from build123d import *

# Parameters (mm, degrees)
SKETCH1_R                                      = 79.248
EXTRUDE1_DEPTH                                 = 3.175
EXTRUDE1_DEPTH_BACK                            = 3.175
SKETCH2_R                                      = 63.5
EXTRUDE2_DEPTH                                 = 10.16
SKETCH4_W                                      = 2.54
SKETCH4_H                                      = 2.3622
SKETCH5_R                                      = 55.88
CUT_EXTRUDE1_DEPTH                             = 10.16
CHAMFER1_SIZE                                  = 1.27
CHAMFER2_SIZE                                  = 0.254
CBORE_FOR_3_SOCKET_HEAD_CAP_SCREW1_D           = 2.794
CBORE_FOR_3_SOCKET_HEAD_CAP_SCREW1_CBORE_D     = 5.15874
CBORE_FOR_3_SOCKET_HEAD_CAP_SCREW1_CBORE_DEPTH = 2.5146
CIRPATTERN1_COUNT                              = 6
F_4_40_TAPPED_HOLE1_D                          = 2.2606
F_4_40_TAPPED_HOLE1_DEPTH                      = 5.08
F_4_40_TAPPED_HOLE1_TIP                        = 0.679152758
M14_CLEARANCE_HOLE1_D                          = 15.5
M14_CLEARANCE_HOLE1_DEPTH                      = 330.2
M14_CLEARANCE_HOLE1_TIP                        = 4.656669797
F_6_32_TAPPED_HOLE1_D                          = 2.7051
F_6_32_TAPPED_HOLE1_DEPTH                      = 4.318
F_6_32_TAPPED_HOLE1_CBORE_D                    = 3.5052
F_6_32_TAPPED_HOLE1_CBORE_DEPTH                = 3.556
F_6_32_TAPPED_HOLE1_TIP                        = 0.81269403
SKETCH21_R                                     = 3.175
SKETCH21_R_2                                   = 1.7526
BOSS_EXTRUDE1_DEPTH                            = 25.4


with BuildPart() as part:
    # Sketch1 → Extrude1 (new body, two sides)
    with BuildSketch(Plane(origin=(0, 0, 0), x_dir=(1, 0, 0), z_dir=(0, 1, 0))) as extrude1_sk:
        Circle(SKETCH1_R)
    extrude(amount=EXTRUDE1_DEPTH)
    extrude(extrude1_sk.sketch, amount=-EXTRUDE1_DEPTH_BACK)

    # Sketch2 → Extrude2 (add)
    with BuildSketch(Plane(origin=(0, 3.175, 0), x_dir=(-1, 0, 0), z_dir=(0, 1, 0))):
        Circle(SKETCH2_R)
    extrude(amount=EXTRUDE2_DEPTH)

    # Sketch4 → Cut-Revolve7 (revolve, cut)
    with BuildSketch(Plane(origin=(0, 0, 0), x_dir=(0, 0, -1), z_dir=(1, 0, 0))):
        with Locations((-62.23, 10.122310801)):
            Rectangle(SKETCH4_W, SKETCH4_H)
        with Locations((-62.23, 6.799968424)):
            Rectangle(SKETCH4_W, SKETCH4_H)
    revolve(axis=Axis((0, -3.175, 0), (0, 1, 0)), mode=Mode.SUBTRACT)

    # Sketch5 → Cut-Extrude1 (cut)
    with BuildSketch(Plane(origin=(0, 13.335, 0), x_dir=(-1, 0, 0), z_dir=(0, 1, 0))):
        Circle(SKETCH5_R)
    extrude(amount=-CUT_EXTRUDE1_DEPTH, mode=Mode.SUBTRACT)

    # Chamfer1
    chamfer1_edges = [part.edges().sort_by_distance(p)[0] for p in [
        (63.5, 13.335, 0),
    ]]
    chamfer(chamfer1_edges, length=CHAMFER1_SIZE)

    # Chamfer2
    chamfer2_edges = [part.edges().sort_by_distance(p)[0] for p in [
        (63.5, 11.303410801, 0),
        (63.5, 8.941210801, 0),
        (63.5, 7.981068424, 0),
        (63.5, 5.618868424, 0),
    ]]
    chamfer(chamfer2_edges, length=CHAMFER2_SIZE)

    # CBORE for _3 Socket Head Cap Screw1 (through all)
    with Locations(Plane(origin=(0, -3.175, 66.675), x_dir=(0, 0, -1), z_dir=(0, -1, 0))):
        with Locations((0, 0)):
            cbore_for_3_socket_head_cap_screw1 = CounterBoreHole(CBORE_FOR_3_SOCKET_HEAD_CAP_SCREW1_D / 2, CBORE_FOR_3_SOCKET_HEAD_CAP_SCREW1_CBORE_D / 2, CBORE_FOR_3_SOCKET_HEAD_CAP_SCREW1_CBORE_DEPTH)

    # CirPattern1: CBORE for _3 Socket Head Cap Screw1 ×6 about axis
    cirpattern1_axis = Axis((0, 0, 0), (0, 1, 0))
    for i in range(1, CIRPATTERN1_COUNT):
        add(cbore_for_3_socket_head_cap_screw1.rotate(cirpattern1_axis, i * 360 / CIRPATTERN1_COUNT), mode=Mode.SUBTRACT)

    # 4-40 Tapped Hole1
    with Locations(Plane(origin=(9.525, 3.175, -36.195), x_dir=(0, 0, 1), z_dir=(0, 1, 0))):
        with Locations((0, 0), (66.675, -26.9875)):
            Hole(F_4_40_TAPPED_HOLE1_D / 2, depth=F_4_40_TAPPED_HOLE1_DEPTH)
            with Locations((0, 0, -(F_4_40_TAPPED_HOLE1_DEPTH + F_4_40_TAPPED_HOLE1_TIP / 2))):  # 118° drill point
                Cone(0, F_4_40_TAPPED_HOLE1_D / 2, F_4_40_TAPPED_HOLE1_TIP, mode=Mode.SUBTRACT)

    # M14 Clearance Hole1
    with Locations(Plane(origin=(-45.367887501, 3.175, 0), x_dir=(0, 0, 1), z_dir=(0, 1, 0))):
        with Locations((0, 0)):
            Hole(M14_CLEARANCE_HOLE1_D / 2, depth=M14_CLEARANCE_HOLE1_DEPTH)
            with Locations((0, 0, -(M14_CLEARANCE_HOLE1_DEPTH + M14_CLEARANCE_HOLE1_TIP / 2))):  # 118° drill point
                Cone(0, M14_CLEARANCE_HOLE1_D / 2, M14_CLEARANCE_HOLE1_TIP, mode=Mode.SUBTRACT)

    # 6-32 Tapped Hole1
    with Locations(Plane(origin=(-19.05, -3.175, 20.574), x_dir=(0, 0, -1), z_dir=(0, -1, 0))):
        with Locations((0, 0), (0, 38.1), (41.148, 38.1), (41.148, 0)):
            CounterBoreHole(F_6_32_TAPPED_HOLE1_D / 2, F_6_32_TAPPED_HOLE1_CBORE_D / 2, F_6_32_TAPPED_HOLE1_CBORE_DEPTH, depth=F_6_32_TAPPED_HOLE1_DEPTH)
            with Locations((0, 0, -(F_6_32_TAPPED_HOLE1_DEPTH + F_6_32_TAPPED_HOLE1_TIP / 2))):  # 118° drill point
                Cone(0, F_6_32_TAPPED_HOLE1_D / 2, F_6_32_TAPPED_HOLE1_TIP, mode=Mode.SUBTRACT)

    # Sketch21 → Boss-Extrude1 (add)
    with BuildSketch(Plane.XZ.offset(3.175)):
        with Locations((19.05, -20.574)):
            Circle(SKETCH21_R)
        with Locations((19.05, -20.574)):
            Circle(SKETCH21_R_2, mode=Mode.SUBTRACT)
        with Locations((-19.05, -20.574)):
            Circle(SKETCH21_R)
        with Locations((-19.05, -20.574)):
            Circle(SKETCH21_R_2, mode=Mode.SUBTRACT)
        with Locations((-19.05, 20.574)):
            Circle(SKETCH21_R)
        with Locations((-19.05, 20.574)):
            Circle(SKETCH21_R_2, mode=Mode.SUBTRACT)
        with Locations((19.05, 20.574)):
            Circle(SKETCH21_R)
        with Locations((19.05, 20.574)):
            Circle(SKETCH21_R_2, mode=Mode.SUBTRACT)
    extrude(amount=BOSS_EXTRUDE1_DEPTH)


solid = part.part
Input: part model. Units: mm. Frame: model coordinates. A direction names the side the tool comes from. Give positions to 0.01 mm unless a question says otherwise; leave off trailing zeros. Order: outer loops, then holes, each group sorted by start corner. A loop starts at its lowest first (then second) coordinate and runs counter-clockwise, first axis right, second up. Notation, with made-up numbers: (75.25, 5) -> (114.25, 5) arc R32 cw to (114.25, 41) -> close; hole circle Ø6 at (87, 31). An arc over 180 degrees is marked (long way). Use one line per item in the form item = value.
1) Line query: probe 1 along X at (y, z) = (9, -0.5); probe 2 along Z at (x, y) = (19.05, -10); probe 3 along Z at (x, y) = (-20.5, -17.5). Output: solid intervals per line, ascending.
Response values:
probe_1 = -60.96 to -55.88, 55.88 to 60.96
probe_2 = -23.75 to -22.33, -18.82 to -17.4, 17.4 to 18.82, 22.33 to 23.75
probe_3 = -23.4 to -21.56, -19.59 to -17.75, 17.75 to 19.59, 21.56 to 23.4
2) Section A-A, the plane y = -26. Return loops of the section in (x, z) (3 decimals).
Response values:
outline = circle Ø6.35 at (-19.05, -20.574); circle Ø6.35 at (-19.05, 20.574); circle Ø6.35 at (19.05, -20.574); circle Ø6.35 at (19.05, 20.574); hole circle Ø3.505 at (-19.05, -20.574); hole circle Ø3.505 at (-19.05, 20.574); hole circle Ø3.505 at (19.05, -20.574); hole circle Ø3.505 at (19.05, 20.574)
3) First-contact query: pin 1 Ø1.8 at (x, z) = (-19.5, -21) entering from -Y; pin 2 Ø3 at (x, z) = (-5, 27.5) entering from +Y (3 decimals); pin 3 Ø8 at (y, z) = (1, 41) entering from -X. Flat tips, straight axial feed; report the tip coordinate or a pass-through.
Response values:
pin_1 = 0.38
pin_2 = 3.175
pin_3 = -70.08
4) Reachability of faces 1 (the flat face through (52, 8.941, -33)), 2 (the flat face through (19, 0.381, -19)), 3 (the flat face through (-59, 3.175, -24)), 4 (the flat face through (-17.68, -28.575, -21.94)), 5 (the cylindrical face through (-37.684, -0.044, 1.009)) from +Z, -Z, +X, -X, +Y, -Y: full face, straight path, thin tool, end or side. Return the list, or none.
Response values:
face_1 = none
face_2 = -Y
face_3 = +Y
face_4 = +Z, -Z, +X, -X, -Y
face_5 = +Y, -Y
5) Mould query, pull axis Y, two halves, no side actions, for faces 6 (the cylindrical face through (7.3, 8.3, 55.4)), 7 (the cylindrical face through (-37.09, 10.14, -48.38)), 8 (the flat face through (20.4, -28.575, 19.2)). Classes: pulls with the +Y half, pulls with the -Y half, needs draft (parallel to the pull), parting line crosses it, or undercut.
Response values:
face_6 = needs draft
face_7 = undercut
face_8 = pulls with the -Y half
